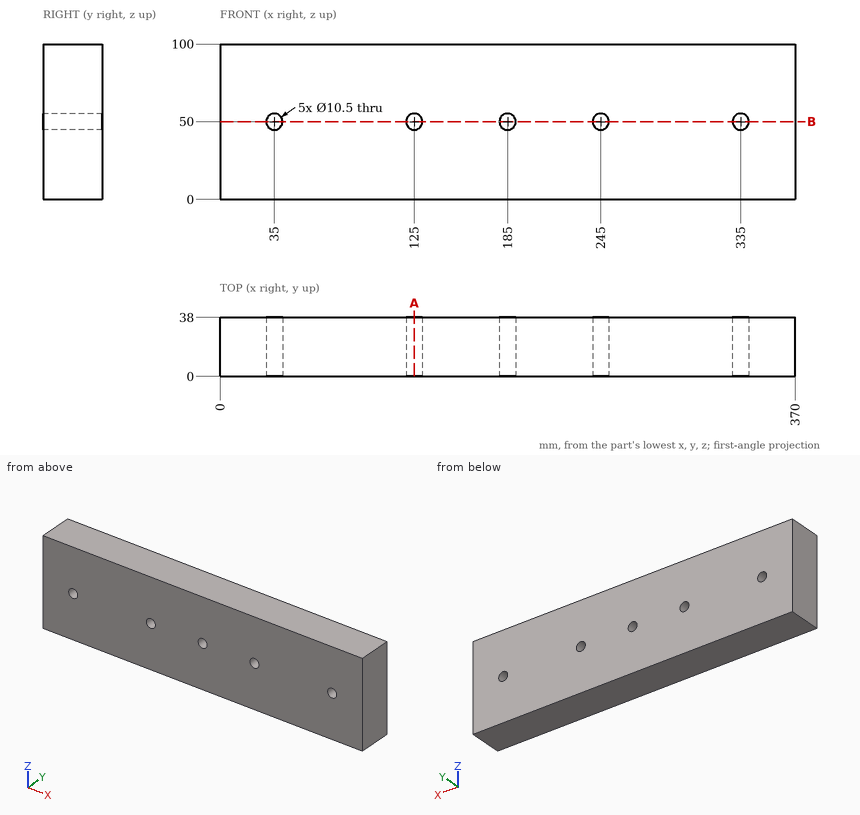
Design review of the part shown in the three views and the two pictorial views. Dimensions are in mm from the part's minimum x, y and z. Give positions to 0.01 mm unless a question says otherwise; leave off trailing zeros. Loops run counter-clockwise (first coordinate to the right, second up) from the corner with the lowest first, then second, coordinate; pieces in that order, holes last. Notation, with made-up numbers: (62.25, 77) -> (78.25, 77) arc R11 cw to (78.25, 83) -> close; hole circle Ø10 at (10.5, -24). An arc over 180 degrees is marked (long way). Answer as a JSON object with one key per item and string values. Group by question number.
Q1. Wall thickness on line 1 along X through (y, z) = (20, 50); line 2 along Z through (x, y) = (245, 25); line 3 along Z through (x, y) = (32.5, 5.5): over which ranges is each line inside the solid? List them lowest first.
Q2. Take a section at B-B (z = 50). Write out the cut boundary in (x, y), plus the area to 3 significant figures.
Q3. Take a section at A-A (x = 125). Write out the cut boundary in (y, z), plus the area to 3 significant figures.
Answer below:
{
 "1": {"line 1": "x = 0 to 29.75, 40.25 to 119.75, 130.25 to 179.75, 190.25 to 239.75, 250.25 to 329.75, 340.25 to 370", "line 2": "z = 0 to 44.75, 55.25 to 100", "line 3": "z = 0 to 45.38, 54.62 to 100"},
 "2": {"outline": "(0, 0) -> (29.75, 0) -> (29.75, 38) -> (0, 38) -> close; (40.25, 0) -> (119.75, 0) -> (119.75, 38) -> (40.25, 38) -> close; (130.25, 0) -> (179.75, 0) -> (179.75, 38) -> (130.25, 38) -> close; (190.25, 0) -> (239.75, 0) -> (239.75, 38) -> (190.25, 38) -> close; (250.25, 0) -> (329.75, 0) -> (329.75, 38) -> (250.25, 38) -> close; (340.25, 0) -> (370, 0) -> (370, 38) -> (340.25, 38) -> close", "area": "12,100 mm2"},
 "3": {"outline": "(0, 0) -> (38, 0) -> (38, 44.75) -> (0, 44.75) -> close; (0, 55.25) -> (38, 55.25) -> (38, 100) -> (0, 100) -> close", "area": "3,400 mm2"}
}
